from build123d import *

# Parameters (mm, degrees)
F1_DEPTH = 24
F2_T     = -2
F3_R     = 8.25
F4_DEPTH = 2
F5_R     = 3
F5_R_2   = 1.5000011027
F6_DEPTH = 22
F8_DEPTH = 10


with BuildPart() as f1:
    # F0 (on Top) → F1 (new body)
    with BuildSketch(Plane.XY):
        with BuildLine():
            ThreePointArc((48.5, 9.5), (47.4748737342, 11.9748737342), (45, 13))
            Line((45, 13), (-45, 13))
            ThreePointArc((-45, 13), (-47.4748737342, 11.9748737342), (-48.5, 9.5))
            Line((-48.5, 9.5), (-48.5, -9.5))
            ThreePointArc((-48.5, -9.5), (-47.4748737342, -11.9748737342), (-45, -13))
            Line((-45, -13), (45, -13))
            ThreePointArc((45, -13), (47.4748737342, -11.9748737342), (48.5, -9.5))
            Line((48.5, -9.5), (48.5, 9.5))
        make_face()
    extrude(amount=F1_DEPTH)

    # F2
    f2_openings = [f1.faces().sort_by_distance(p)[0] for p in [
        (0, 0, 24),
    ]]
    offset(amount=F2_T, openings=f2_openings)

    # F3 (on face) → F4 (cut, through all)
    with BuildSketch(Plane(origin=(0, 0, 0), x_dir=(1, 0, 0), z_dir=(0, 0, -1))):
        with Locations((13.5, -2.15)):
            Circle(F3_R)
    extrude(amount=-F4_DEPTH, mode=Mode.SUBTRACT)

    # F5 (on face) → F6 (join, through all)
    with BuildSketch(Plane.XY.offset(2)):
        with Locations((-45, 9.5)):
            Circle(F5_R)
        with Locations((-45, 9.5)):
            Circle(F5_R_2, mode=Mode.SUBTRACT)
        with Locations((45, 9.5)):
            Circle(F5_R)
        with Locations((45, 9.5)):
            Circle(F5_R_2, mode=Mode.SUBTRACT)
        with Locations((-45, -9.5)):
            Circle(F5_R)
        with Locations((-45, -9.5)):
            Circle(F5_R_2, mode=Mode.SUBTRACT)
        with Locations((45, -9.5)):
            Circle(F5_R)
        with Locations((45, -9.5)):
            Circle(F5_R_2, mode=Mode.SUBTRACT)
    extrude(amount=F6_DEPTH)

    # F7 (on face) → F8 (cut)
    with BuildSketch(Plane.YZ.offset(48.5)):
        Polygon((9.5, 19), (-9.5, 19), (-9.5, 12), (-2.5, 12), (-2.5, 10.7), (1.5, 10.7), (1.5, 12), (9.5, 12), align=None)
    extrude(amount=-F8_DEPTH, mode=Mode.SUBTRACT)


solid = f1.part
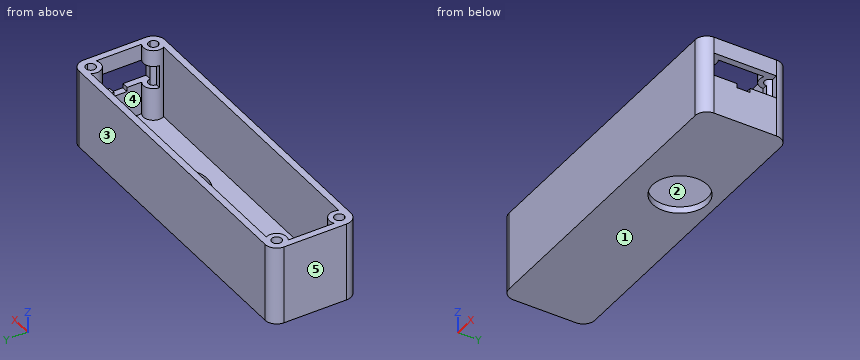
Geometry check sheet. Reference: the model listing, model coordinates, mm. Face numbers are marked on the shaded views. A direction names the side the tool comes from. Round coordinates to 2 decimals unless told otherwise and drop trailing zeros. Write each loop counter-clockwise with the first axis right and the second up, starting at its lowest first coordinate (ties: lowest second). Pieces come first, ordered by that corner, then holes.
Item 1: Go/stop test with flat-tipped pins: pin 1 Ø0.9 at (x, y) = (45.5, -9) entering from +Z; pin 2 Ø2.5 at (x, y) = (45.5, 10) entering from +Z; pin 3 Ø1.6 at (x, z) = (48, 15) entering from -Y. Record where each tip stops, or that it passes through.
Determined:
pin 1: stops at z = 2
pin 2: stops at z = 24
pin 3: stops at y = -12.22
Item 2: Section check C-C (z = 14). Record the boundary of the cut face in (x, y), plus the area to 3 significant figures.
Determined:
outline: (-48.5, -9.5) arc R3.5 ccw to (-45, -13) - (45, -13) arc R3.5 ccw to (48.5, -9.5) - (46.5, -9.5) arc R1.5 cw to (45, -11) arc R1.5 cw to (43.5, -9.5) - (42, -9.5) arc R3 ccw to (42.4, -11) - (-42.4, -11) arc R3 ccw to (-46.5, -6.9) - (-46.5, 6.9) arc R3 ccw to (-42.4, 11) - (42.4, 11) arc R3 ccw to (42, 9.5) - (43.5, 9.5) arc R1.5 cw to (45, 11) arc R1.5 cw to (46.5, 9.5) - (48.5, 9.5) arc R3.5 ccw to (45, 13) - (-45, 13) arc R3.5 ccw to (-48.5, 9.5) - close; hole (-46.5, -9.5) arc R1.5 ccw to (-45, -11) arc R1.5 ccw (long way) to start; hole (-46.5, 9.5) arc R1.5 ccw (long way) to (-45, 11) arc R1.5 ccw to start
area: 455 mm2
Item 3: Mould release check, pull along Y, two halves, no side actions. Record for the marked faces 1, 2 and 3: +Y half, -Y half, draft (parallel to the pull), parting line (faces both ways), or undercut.
Determined:
face 1: draft
face 2: undercut
face 3: +Y half
Item 4: Section check A-A (x = 13.5). Record the boundary of the cut face in (y, z).
Determined:
outline: (-13, 0) - (-6.1, 0) - (-6.1, 2) - (-11, 2) - (-11, 24) - (-13, 24) - close; (10.4, 0) - (13, 0) - (13, 24) - (11, 24) - (11, 2) - (10.4, 2) - close
Item 5: Section check B-B (y = 0.5). Record the boundary of the cut face in (x, z).
Determined:
outline: (-48.5, 0) - (5.42, 0) - (5.42, 2) - (-46.5, 2) - (-46.5, 24) - (-48.5, 24) - close; (21.58, 0) - (48.5, 0) - (48.5, 10.7) - (46.5, 10.7) - (46.5, 2) - (21.58, 2) - close; (46.5, 19) - (48.5, 19) - (48.5, 24) - (46.5, 24) - close
Item 6: Material ranges on line 1 along Y through (x, z) = (45, 10); line 2 along X through (y, z) = (-9.5, 7.5); line 3 along Y through (x, z) = (44, 22), recorded low to high.
Determined:
line 1: y = -13 to -11, -8 to -6.5, 6.5 to 8, 11 to 13
line 2: x = -48.5 to -46.5, -43.5 to -42, 42 to 43.5, 46.5 to 48.5
line 3: y = -13 to -10.62, -8.38 to -6.67, 6.67 to 8.38, 10.62 to 13
Item 7: Access from +Z, -Z, +X, -X, +Y, -Y to the whole of each face (thin tool, end or side, straight path). Record for the marked faces 4 and 5.
Determined:
face 4: +Z
face 5: +Z, -Z, -X, +Y, -Y
